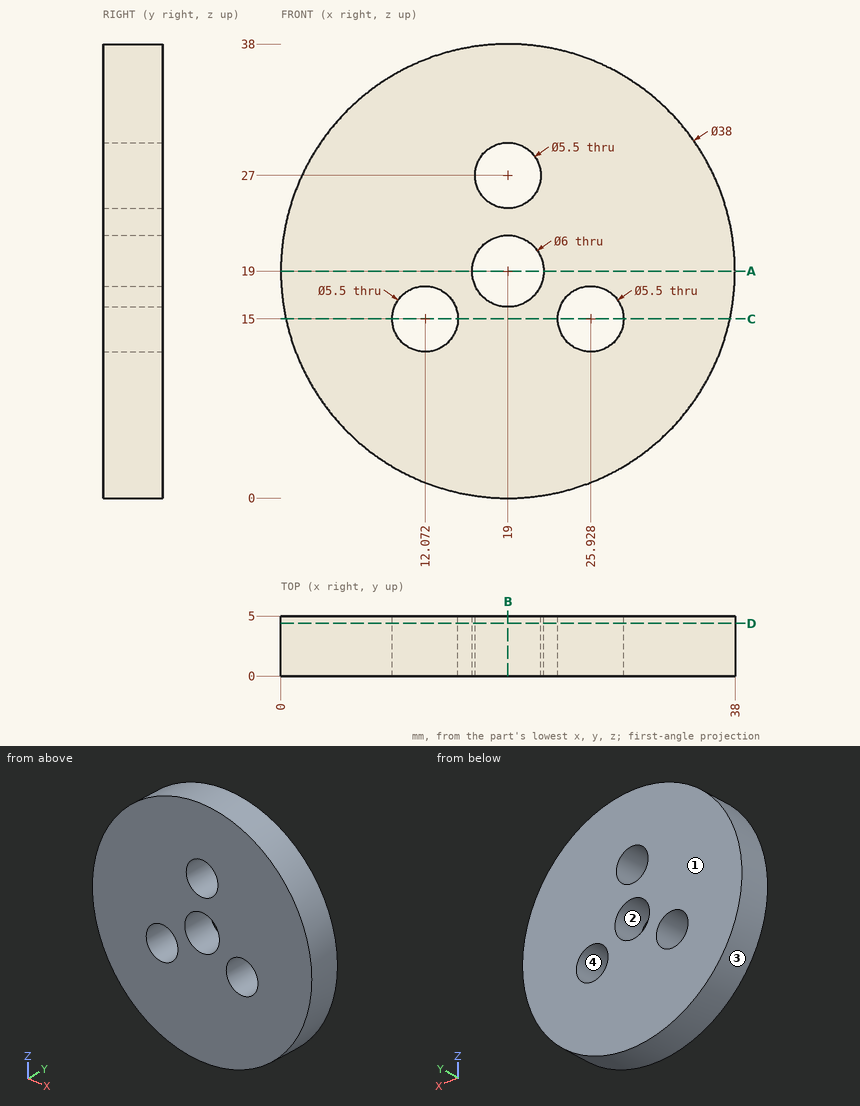
Drawing for the job (mm, zero at the part's lowest x, y, z). Round coordinates to 2 decimals unless told otherwise and drop trailing zeros. Order: outer loops, then holes, each group sorted by start corner. A loop starts at its lowest first (then second) coordinate and runs counter-clockwise, first axis right, second up.
Item 1: Probe line 1 along Z through (x, y) = (19, 2.4); line 2 along X through (y, z) = (3.5, 21.5) (1 decimal); line 3 along Z through (x, y) = (26, 4.75). List the from-to ranges inside material, lowest first.
Item 2: Saw through at D-D on y = 4.4. Write the cut outline in (x, z).
Item 3: Mould opens along Z. For the marked faces 1, 2, 3 and 4 say: pulls with the +Z half, pulls with the -Z half, needs draft (parallel to the pull), parting line crosses it, or undercut.
Item 4: Saw through at A-A on z = 19. Write the cut outline in (x, y), then the cut area to 3 significant figures.
Item 5: Pin check, flat tips, straight feed: pin 1 (1.5 mm diameter, centred on x = 22, y = 3, fed in from +Z); pin 2 (1 mm diameter, centred on y = 2.5, z = 32.5, fed in from -X); pin 3 (2 mm diameter, centred on y = 0.5, z = 5, fed in from +X). Stop position of each tip, or through.
Item 6: Saw through at C-C on z = 15. Write the cut outline in (x, y).
Item 7: Saw through at B-B on x = 19. Write the cut outline in (y, z), then the cut area to 4 significant figures.
Reported:
1. line 1: z = 0 to 16, 22 to 24.25, 29.75 to 38
1. line 2: x = 0.2 to 17.3, 20.7 to 37.8
1. line 3: z = 1.34 to 12.25, 17.75 to 36.66
2. outline: circle Ø38 at (19, 19); hole circle Ø5.5 at (12.07, 15); hole circle Ø6 at (19, 19); hole circle Ø5.5 at (19, 27); hole circle Ø5.5 at (25.93, 15)
3. face 1: needs draft
3. face 2: undercut
3. face 3: parting line crosses it
3. face 4: undercut
4. outline: (0, 0) - (16, 0) - (16, 5) - (0, 5) - close; (22, 0) - (38, 0) - (38, 5) - (22, 5) - close
4. area: 160 mm2
5. pin 1: stops at z = 37.87
5. pin 2: stops at x = 5.14
5. pin 3: stops at x = 32.86
6. outline: (0.43, 0) - (9.32, 0) - (9.32, 5) - (0.43, 5) - close; (14.82, 0) - (23.18, 0) - (23.18, 5) - (14.82, 5) - close; (28.68, 0) - (37.57, 0) - (37.57, 5) - (28.68, 5) - close
7. outline: (0, 0) - (5, 0) - (5, 16) - (0, 16) - close; (0, 22) - (5, 22) - (5, 24.25) - (0, 24.25) - close; (0, 29.75) - (5, 29.75) - (5, 38) - (0, 38) - close
7. area: 132.5 mm2
